Geometry check sheet. Reference: the model listing, model coordinates, mm. Face numbers are marked on the shaded views. A direction names the side the tool comes from. Give positions to 0.01 mm unless a question says otherwise; leave off trailing zeros. Order: outer loops, then holes, each group sorted by start corner. A loop starts at its lowest first (then second) coordinate and runs counter-clockwise, first axis right, second up. Notation, with made-up numbers: M 81,89.25 L 118,89.25 A35 ccw 118,127.25 Z; hole C 2.5,13 d9. An arc over 180 degrees is marked long. Answer as a JSON object with one key per item and string values. Group by question number.
from build123d import *


with BuildPart() as f1:
    # F0 (on Right) → F1 (revolve)
    with BuildSketch(Plane.YZ):
        with BuildLine():
            Line((0, 3.75), (0, 0))
            Line((0, 0), (18.8, 0))
            Line((18.8, 0), (18.8, 3.75))
            ThreePointArc((18.8, 3.75), (18.726777, 3.926777), (18.55, 4))
            Line((18.55, 4), (16.4, 4))
            Line((16.4, 4), (16.4, 3.25))
            Line((16.4, 3.25), (15.4, 3.25))
            Line((15.4, 3.25), (15.4, 4.6))
            Line((15.4, 4.6), (4.4, 4.6))
            Line((4.4, 4.6), (4.4, 3.25))
            Line((4.4, 3.25), (2.4, 3.25))
            Line((2.4, 3.25), (2.4, 4))
            Line((2.4, 4), (0.25, 4))
            ThreePointArc((0.25, 4), (0.073223, 3.926777), (0, 3.75))
        make_face()
    revolve(axis=Axis((0, 9.4, 0), (0, 1, 0)))


solid = f1.part
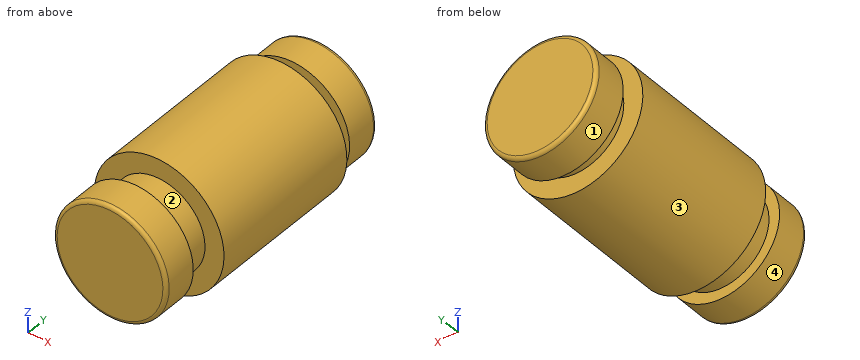
1. Access from +Z, -Z, +X, -X, +Y, -Y to the whole of each face (thin tool, end or side, straight path). Record for the marked faces 1, 2, 3 and 4.
2. Cross-section at A-A (z = 0). Record the cut outline in (x, y).
3. Depth check by flat-ended pin: pin 1 (1.5 mm diameter, centred on y = 7.5, z = -3.5, fed in from -X); pin 2 (2 mm diameter, centred on x = 3.5, y = 13, fed in from -Z); pin 3 (3 mm diameter, centred on y = 4.5, z = 2.5, fed in from +X). Enter the tip coordinate at first touch or a pass-through.
4. Cross-section at B-B (x = 0). Record the cut outline in (y, z), and give its area (3 significant figures).
5. Thickness scan on line 1 along Y through (x, z) = (2, 3); line 2 along Y through (x, z) = (4.25, 0); line 3 along X through (y, z) = (2.5, -2.5). Record the ranges inside material, lowest first. Write a range as [from, to].
6. Cross-section at D-D (x = -3.5). State how many separate pieces and enclosed holes the cut face has, and give its area (3 significant figures).
7. Cross-section at C-C (y = 12.75). Record the cut outline in (x, z).
Report:
{
 "1": {"face 1": "+Y", "face 2": "none", "face 3": "+Y, -Y", "face 4": "-Y"},
 "2": {"outline": "M -4.6,4.4 L -3.25,4.4 L -3.25,2.4 L -4,2.4 L -4,0.25 A0.25 ccw -3.75,0 L 3.75,0 A0.25 ccw 4,0.25 L 4,2.4 L 3.25,2.4 L 3.25,4.4 L 4.6,4.4 L 4.6,15.4 L 3.25,15.4 L 3.25,16.4 L 4,16.4 L 4,18.55 A0.25 ccw 3.75,18.8 L -3.75,18.8 A0.25 ccw -4,18.55 L -4,16.4 L -3.25,16.4 L -3.25,15.4 L -4.6,15.4 Z"},
 "3": {"pin 1": "stops at x = -3.69", "pin 2": "stops at z = -3.86", "pin 3": "stops at x = 4.49"},
 "4": {"outline": "M 0,-3.75 A0.25 ccw 0.25,-4 L 2.4,-4 L 2.4,-3.25 L 4.4,-3.25 L 4.4,-4.6 L 15.4,-4.6 L 15.4,-3.25 L 16.4,-3.25 L 16.4,-4 L 18.55,-4 A0.25 ccw 18.8,-3.75 L 18.8,3.75 A0.25 ccw 18.55,4 L 16.4,4 L 16.4,3.25 L 15.4,3.25 L 15.4,4.6 L 4.4,4.6 L 4.4,3.25 L 2.4,3.25 L 2.4,4 L 0.25,4 A0.25 ccw 0,3.75 Z", "area": "159 mm2"},
 "5": {"line 1": "y = [0, 2.4], [4.4, 15.4], [16.4, 18.8]", "line 2": "y = [4.4, 15.4]", "line 3": "x = [-2.08, 2.08]"},
 "6": {"separate pieces": "3", "enclosed holes": "0", "area": "84.1 mm2"},
 "7": {"outline": "C 0,0 d9.2"}
}
